Design review of the part built by this model. Coordinates are the model's own, in mm. Give positions to 0.01 mm unless a question says otherwise; leave off trailing zeros. Loops run counter-clockwise (first coordinate to the right, second up) from the corner with the lowest first, then second, coordinate; pieces in that order, holes last. Notation, with made-up numbers: (18.5, -39.75) -> (52.5, -39.75) arc R18 cw to (52.5, -18.75) -> close; hole circle Ø5 at (16.25, 13). An arc over 180 degrees is marked (long way). Use a Markdown table: item, result. Add a question column.
1. Add section C-C (y = 163). State the section outline as (x, z) points, and give its area (3 significant figures).
2. Add section A-A (y = 213). State the section outline as (x, z) points, and give its area (3 significant figures).
3. Add section D-D (x = 552). Count the separate pieces of the cut face and the enclosed holes in it, and give its area (3 significant figures).
4. Add section B-B (x = 600.5). State the section outline as (y, z) points.
5. For pin 1 Ø12 at (x, y) = (594.5, 234.5) entering from +Z; pin 2 Ø8 at (x, y) = (692.5, 69) entering from +Z; pin 3 Ø12 at (x, y) = (510, 68) entering from -Z, all flat-tipped, find the tip position at first contact; note any pin that passes through.
6. To check wall thickness, follow line 1 (Z direction, x = 650.5, y = 87); line 2 (Z direction, x = 490, y = 243). State the ranges of each line that lie inside material, in increasing order.
```python
from build123d import *

# Parameters (mm, degrees)
SKETCH1_W                      = 278.13
SKETCH1_H                      = 251.191235252
BOSS_EXTRUDE1_DEPTH            = 6.35
DRAFT1_ANGLE                   = -12.5
HOLE1_D                        = 28.575
HOLE1_DEPTH                    = 59.131528827
F_7_0_201_DIAMETER_HOLE1_D     = 5.1054
F_7_0_201_DIAMETER_HOLE1_DEPTH = 59.131528827
CUT_EXTRUDE1_DEPTH             = 643.237238264
CUT_EXTRUDE1_DEPTH_BACK        = 643.237238264
SKETCH6_R                      = 2.5527
BOSS_EXTRUDE2_DEPTH            = 1.27


with BuildPart() as part:
    # Sketch1 → Boss-Extrude1 (new body)
    with BuildSketch(Plane(origin=(158.268774626, 0, 713.904307571), x_dir=(0, 1, 0), z_dir=(0.2164396139381031, 0, 0.9762960071199334))):
        with Locations((145.415, -448.825686245)):
            Rectangle(SKETCH1_W, SKETCH1_H)
    extrude(amount=-BOSS_EXTRUDE1_DEPTH)

    # Draft1
    draft1_faces = [part.faces().sort_by_distance(p)[0] for p in [
        (473.149804226, 145.415, 640.844776483),
    ]]
    draft(draft1_faces, Plane(origin=(158.268774626, 0, 713.904307571), x_dir=(0.9762960071199334, 0, -0.2164396139381031), z_dir=(0.21643961393810307, 0, 0.9762960071199333)), DRAFT1_ANGLE)

    # Hole1
    with Locations(Plane(origin=(158.268774626, 0, 713.904307571), x_dir=(0.9762960071199339, 0, -0.21643961393810046), z_dir=(0.21643961393810046, 0, 0.9762960071199339))):
        with Locations((348.630068619, 69.85), (508.166081715, 57.15), (508.166081715, 234.95), (348.630068619, 222.25), (414.112652808, 42.099584365), (414.112652808, 250.000415635)):
            Hole(HOLE1_D / 2, depth=HOLE1_DEPTH)

    # #7 (0.201) Diameter Hole1
    with Locations(Plane(origin=(158.268774626, 0, 713.904307571), x_dir=(0.9762960071199334, 0, -0.21643961393810307), z_dir=(0.21643961393810304, 0, 0.9762960071199333))):
        with Locations((461.529064979, 273.05), (512.329064979, 273.05), (563.129064979, 273.05), (537.729064979, 273.05), (486.929064979, 273.05), (368.368874158, 273.05), (461.529064979, 19.05), (486.929064979, 19.05), (512.329064979, 19.05), (537.729064979, 19.05), (563.129064979, 19.05), (368.368874158, 19.05), (342.968874158, 19.05), (432.07316505, 24.139072123), (432.07316505, 60.060096607), (396.152140566, 24.139072123), (396.152140566, 60.060096607), (432.07316505, 267.960927877), (396.152140566, 267.960927877), (432.07316505, 232.039903393), (396.152140566, 232.039903393), (342.968874158, 273.05)):
            Hole(F_7_0_201_DIAMETER_HOLE1_D / 2, depth=F_7_0_201_DIAMETER_HOLE1_DEPTH)

    # Sketch6 → Cut-Extrude1 (cut, two sides: drawn at the far end of the back side and taken through both)
    with BuildSketch(Plane(origin=(158.268774626, 0, 713.904307571), x_dir=(0.9762960071199334, 0, -0.21643961393810307), z_dir=(0.21643961393810304, 0, 0.9762960071199333)).offset(-CUT_EXTRUDE1_DEPTH_BACK)):
        with Locations((388.712652808, 250.000415635)):
            Circle(SKETCH6_R)
        with Locations((414.112652808, 275.400415635)):
            Circle(SKETCH6_R)
        with Locations((439.512652808, 250.000415635)):
            Circle(SKETCH6_R)
        with Locations((414.112652808, 224.600415635)):
            Circle(SKETCH6_R)
        with Locations((388.712652808, 42.099584365)):
            Circle(SKETCH6_R)
        with Locations((414.112652808, 67.499584365)):
            Circle(SKETCH6_R)
        with Locations((439.512652808, 42.099584365)):
            Circle(SKETCH6_R)
        with Locations((414.112652808, 16.699584365)):
            Circle(SKETCH6_R)
    extrude(amount=CUT_EXTRUDE1_DEPTH + CUT_EXTRUDE1_DEPTH_BACK, mode=Mode.SUBTRACT)

    # Sketch7 → Boss-Extrude2 (add)
    with BuildSketch(Plane(origin=(0, 284.48, 0), x_dir=(1, 0, 0), z_dir=(0, 1, 0))):
        Polygon((473.837, -637.44034139), (473.837, -643.944516305), (719.074, -589.576782323), (717.699608451, -583.377302678), align=None)
    extrude(amount=BOSS_EXTRUDE2_DEPTH)


solid = part.part
```
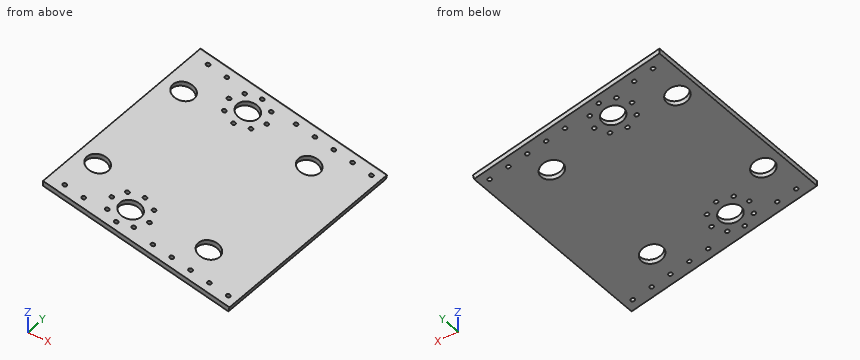
Taken from the geometry:
| question | item | result |
|---|---|---|
| 1 | outline | (473.84, 637.44) -> (717.7, 583.38) -> (719.07, 589.58) -> (473.84, 643.94) -> close |
| 1 | area | 1,590 mm^2 |
| 2 | outline | (473.84, 637.44) -> (486.63, 634.6) -> (488, 640.8) -> (473.84, 643.94) -> close; (507.89, 629.89) -> (717.7, 583.38) -> (719.07, 589.58) -> (509.27, 636.09) -> close |
| 2 | area | 1,450 mm^2 |
| 3 | separate pieces | 3 |
| 3 | enclosed holes | 0 |
| 3 | area | 1,560 mm^2 |
| 4 | outline | (6.35, 609.36) -> (285.75, 609.36) -> (285.75, 615.86) -> (6.35, 615.86) -> close |
| 5 | pin 1 | stops at z = 618.52 |
| 5 | pin 2 | stops at z = 596.35 |
| 5 | pin 3 | stops at z = 628.09 |
| 6 | line 1 | z = 598.28 to 604.78 |
| 6 | line 2 | z = 633.86 to 640.36 |
